Verification items for this drawing (mm, ordinates from the low corner). Coordinates: 2 decimals unless noted, no trailing zeros. Loops run counter-clockwise (first coordinate to the right, second up) from the corner with the lowest first, then second, coordinate; pieces in that order, holes last. Notation, with made-up numbers: M 78,-36.75 L 134,-36.75 A15 ccw 134,-30.75 Z; hole C 25.25,86.5 d2. An arc over 180 degrees is marked long. Write each question's results on one line, items separated by ' | '. Start each with the question number.
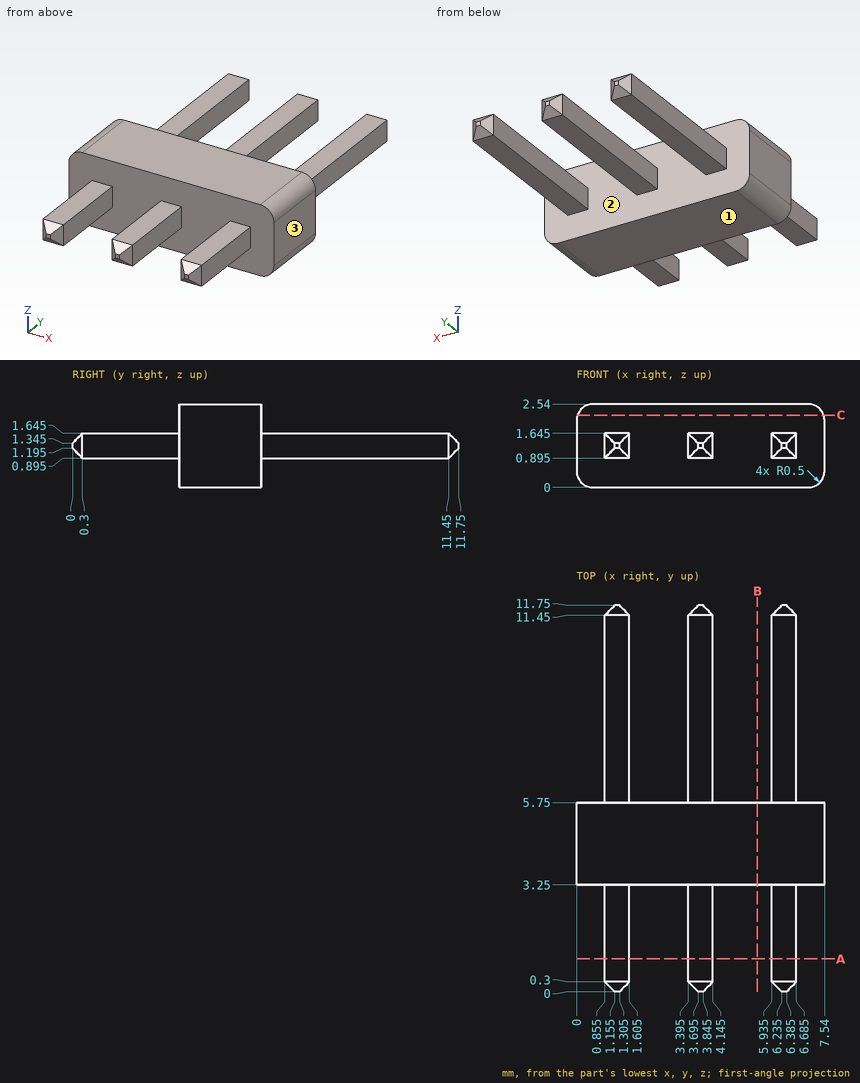
Item 1: Depth check by flat-ended pin: P1, Ø0.8, axis at y = 2, z = 1.5, coming from the -X side (3 decimals); P2, Ø0.8, axis at x = 1.5, y = 1.5, coming from the +Z side (3 decimals); P3, Ø1, axis at x = 5, z = 1.5, coming from the -Y side. Enter the tip coordinate at first touch or a pass-through.
Item 2: Section check A-A (y = 1). Record the cut outline in (x, z) (3 decimals).
Item 3: Section check C-C (z = 2.2). Record the cut outline in (x, y).
Item 4: Section check B-B (x = 5.5). Record the cut outline in (y, z).
Item 5: Release check for a two-part mould opening along X. For the marked faces 1, 2 and 3 record: +X half, -X half, draft (parallel to the pull), parting line (faces both ways), or undercut.
Item 6: Thickness scan on line 1 (X direction, y = 1.5, z = 1.6) (3 decimals); line 2 (Y direction, x = 3.25, z = 1.45); line 3 (Z direction, x = 3.5, y = 7.5) (3 decimals). Record the ranges inside material, lowest first.
Computed values:
1) P1: stops at x = 0.855 | P2: stops at z = 1.645 | P3: stops at y = 3.25
2) outline: M 0.855,0.895 L 1.605,0.895 L 1.605,1.645 L 0.855,1.645 Z; M 3.395,0.895 L 4.145,0.895 L 4.145,1.645 L 3.395,1.645 Z; M 5.935,0.895 L 6.685,0.895 L 6.685,1.645 L 5.935,1.645 Z
3) outline: M 0.03,3.25 L 7.51,3.25 L 7.51,5.75 L 0.03,5.75 Z
4) outline: M 3.25,0 L 5.75,0 L 5.75,2.54 L 3.25,2.54 Z
5) face 1: draft | face 2: undercut | face 3: +X half
6) line 1: x = 0.855 to 1.605, 3.395 to 4.145, 5.935 to 6.685 | line 2: y = 3.25 to 5.75 | line 3: z = 0.895 to 1.645
